Autodesk Inventor part; units mm, degrees
ref_plane "YZ Plane" through (0, 0, 0) normal (1, 0, 0) x (0, 1, 0)
ref_plane "XZ Plane" through (0, 0, 0) normal (0, 1, 0) x (-1, 0, 0)
ref_plane "XY Plane" through (0, 0, 0) normal (0, 0, 1) x (1, 0, 0)
sketch "Skizze1" plane through (0, 0, 0) normal (1, 0, 0) x (0, 1, 0)
  line L0 (0, 0) -> (60, 0)
  line L1 (60, 0) -> (60, -60)
  line L2 (60, -60) -> (0, -60)
  line L3 (0, -60) -> (0, 0)
  line L4 (0, -30) -> (60, -30) construction
  line L5 (30, 0) -> (30, -60) construction
  circle A0 centre (30, -30) radius 29
  line L6 (0, -5) -> (60, -5) construction
  line L7 (60, -55) -> (0, -55) construction
  line L8 (5, 0) -> (5, -60) construction
  line L9 (55, -60) -> (55, 0) construction
  circle A1 centre (55, -5) radius 2.25
  circle A2 centre (55, -55) radius 2.25
  circle A3 centre (5, -55) radius 2.25
  circle A4 centre (5, -5) radius 2.25
  dimension "d0" = 60
  dimension "d1" = 60
  dimension "d2" = 58
  dimension "d3" = 5
  dimension "d4" = 5
  dimension "d5" = 5
  dimension "d6" = 5
  dimension "d7" = 4.5
  dimension "d8" = 4.5
  dimension "d9" = 4.5
  dimension "d10" = 4.5
extrude "Extrusion1" add sketch "Skizze1" against normal blind 3
sketch "Skizze2" plane through (0, 0, -60) normal (0, -1, 0) x (1, 0, 0)
  line L0 (0, 60) -> (-13, 60)
  line L1 (-13, 60) -> (-13, 0)
  line L2 (-13, 0) -> (0, 0)
  line L3 (-1.5, 60) -> (-1.5, 0) construction
  line L4 (0, 60) -> (-3, 60)
  line L5 (0, 60) -> (0, 0)
  line L6 (-10.5, 0) -> (-10.5, 60) construction
  line L7 (5, 57.5) -> (-13, 57.5) construction
  line L8 (5, 2.5) -> (-13, 2.5) construction
  circle A0 centre (-10.5, 57.5) radius 1.75
  circle A1 centre (-10.5, 2.5) radius 1.75
  line L9 (0, 60) -> (0, 0)
  point P0 (-3, 0)
  dimension "d13" = 13
  dimension "d14" = 1.5
  dimension "d17" = 2.5
  dimension "d18" = 2.5
  dimension "d19" = 2.5
  dimension "d21" = 3.5
  dimension "d23" = 3.5
fillet "Rundung1" radius 2 2 edges at (-1.5, 60, -60) (-1.5, 60, 0)
extrude "Extrusion4" add sketch "Skizze2" along normal blind 3
fillet "Rundung2" radius 2 2 edges at (-13, -1.5, 0) (-13, -1.5, -60)
properties part number "Halter_Lüfter"
Work out the finished part from the listing and answer in its coordinate system (mm). A direction names the side the tool comes from. Round coordinates to 2 decimals unless told otherwise and drop trailing zeros. Write each loop counter-clockwise with the first axis right and the second up, starting at its lowest first coordinate (ties: lowest second). Pieces come first, ordered by that corner, then holes. Notation, with made-up numbers: (36, 77) - (70, 77) arc R21 ccw to (70, 105) - close; hole circle Ø10 at (18.5, 17). An arc over 180 degrees is marked (long way). Answer in a Markdown table with one row per item. Add a question column.
1. A cutting plane is placed at C-C, the plane z = -55. Determine the outline of the cut face in (x, y), and give its area (3 significant figures).
2. A cutting plane is placed at D-D, the plane y = 5. Determine the outline of the cut face in (x, z), and give its area (3 significant figures).
3. A cutting plane is placed at A-A, the plane z = -30. Determine the outline of the cut face in (x, y), and give its area (3 significant figures).
4. The mould has two halves that part along Y. Classify faces 3 (the cylindrical face through (-1.479, 52.752, -54.901)), 4 (the flat face through (-8, 0, -30)), 5 (the cylindrical face through (-8.883, -1.479, -1.83)), 6 (the cylindrical face through (-1.479, 6.21, -53.103)): +Y half, -Y half, draft (parallel to the pull), parting line (faces both ways), or undercut.
5. Given pin 1 (6 mm diameter, centred on y = 55, z = -55, fed in from +X); pin 2 (10 mm diameter, centred on y = 15.5, z = -8, fed in from -X), each flat-ended and moving along its own axis, determine where each tip first touches the part or whether it passes through.
6. A cutting plane is placed at B-B, the plane y = 30. Determine the outline of the cut face in (x, z).
7. For faces 1 (the flat face through (-3, 5, -14)), 2 (the cylindrical face through (-1.48, 6.99, -47.65)), determine the directions among +Z, -Z, +X, -X, +Y, -Y from which every point of the face is accessible in a straight line to the end or side of a thin tool.
8. Find the intervals of material crossed by line 1 along Z through (x, y) = (-0.95, 5); line 2 along X through (y, z) = (54, -50), in increasing order. Write a range as from..to.
Worked out:
| question | item | result |
|---|---|---|
| 1 | outline | (-13, -3) - (0, -3) - (0, 2.75) - (-3, 2.75) - (-3, 0) - (-13, 0) - close; (-3, 7.25) - (0, 7.25) - (0, 15.3) - (-3, 15.3) - close; (-3, 44.7) - (0, 44.7) - (0, 52.75) - (-3, 52.75) - close; (-3, 57.25) - (0, 57.25) - (0, 60) - (-3, 60) - close |
| 1 | area | 104 mm^2 |
| 2 | outline | (-3, -60) - (0, -60) - (0, -57.25) - (-3, -57.25) - close; (-3, -52.75) - (0, -52.75) - (0, -44.7) - (-3, -44.7) - close; (-3, -15.3) - (0, -15.3) - (0, -7.25) - (-3, -7.25) - close; (-3, -2.75) - (0, -2.75) - (0, 0) - (-3, 0) - close |
| 2 | area | 64.8 mm^2 |
| 3 | outline | (-13, -3) - (0, -3) - (0, 1) - (-3, 1) - (-3, 0) - (-13, 0) - close; (-3, 59) - (0, 59) - (0, 60) - (-3, 60) - close |
| 3 | area | 45.0 mm^2 |
| 4 | face 3 | undercut |
| 4 | face 4 | +Y half |
| 4 | face 5 | draft |
| 4 | face 6 | undercut |
| 5 | pin 1 | x = 0 |
| 5 | pin 2 | x = -3 |
| 6 | outline | (-3, -60) - (0, -60) - (0, -59) - (-3, -59) - close; (-3, -1) - (0, -1) - (0, 0) - (-3, 0) - close |
| 7 | face 1 | +Z, -Z, -X, +Y |
| 7 | face 2 | +X, -X |
| 8 | line 1 | -60..-57.25, -52.75..-44.7, -15.3..-7.25, -2.75..0 |
| 8 | line 2 | -3..0 |
